For this review, use the dimensioned drawing (mm, ordinates from the lowest corner) and the shaded views. A direction names the side the tool comes from. Round coordinates to 2 decimals unless told otherwise and drop trailing zeros. Loops run counter-clockwise (first coordinate to the right, second up) from the corner with the lowest first, then second, coordinate; pieces in that order, holes last. Notation, with made-up numbers: (-11, 9.5) -> (21, 9.5) arc R23 cw to (21, 32.5) -> close; hole circle Ø3 at (49.5, 30.5). An arc over 180 degrees is marked (long way). Write each question's results on one line, items separated by ' | '.
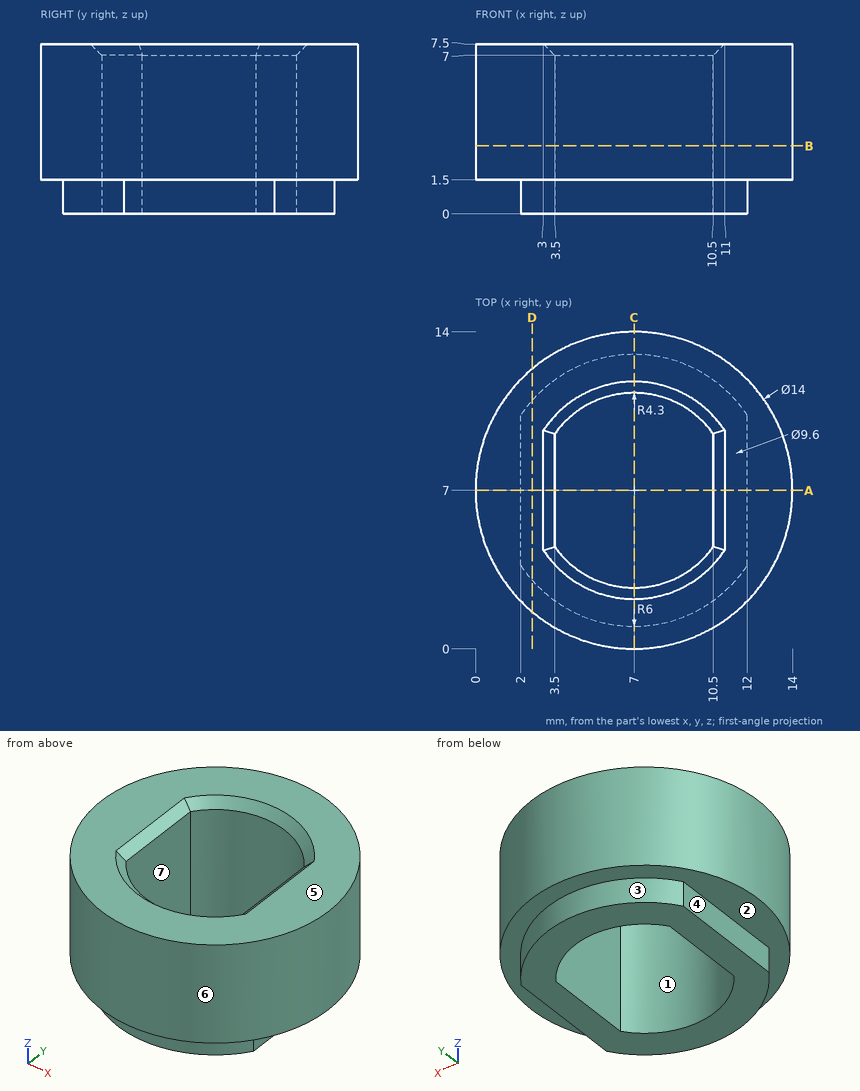
1. Consider section A-A (y = 7). State the section outline as (x, z) points.
Values found:
outline: (0, 1.5) -> (2, 1.5) -> (2, 0) -> (3.5, 0) -> (3.5, 7) -> (3, 7.5) -> (0, 7.5) -> close; (10.5, 0) -> (12, 0) -> (12, 1.5) -> (14, 1.5) -> (14, 7.5) -> (11, 7.5) -> (10.5, 7) -> close
2. For pin 1 (1.5 mm diameter, centred on y = 8, z = 3, fed in from +X); pin 2 (1.6 mm diameter, centred on y = 6.5, z = 0.5, fed in from -X); pin 3 (4 mm diameter, centred on x = 9.5, z = 6, fed in from +Y), all flat-tipped, find the tip position at first contact; note any pin that passes through.
Values found:
pin 1: stops at x = 14 | pin 2: stops at x = 2 | pin 3: stops at y = 13.98
3. Draft analysis for pull direction X (two halves, no side actions). For the marked faces 4, 5, 6 and 7, state which applies: released by +X, released by -X, zero draft, split by the parting line, or undercut.
Values found:
face 4: released by -X | face 5: zero draft | face 6: split by the parting line | face 7: undercut
4. To check wall thickness, follow probe 1 along X at (y, z) = (5.75, 1.25); probe 2 along Z at (x, y) = (1, 3.5); probe 3 along X at (y, z) = (12, 1.25). State the ranges of each line that lie inside material, in increasing order.
Values found:
probe 1: x = 2 to 3.5, 10.5 to 12 | probe 2: z = 1.5 to 7.5 | probe 3: x = 3.68 to 10.32
5. Tool access review of the marked faces 1, 2 and 3: name each direction out of +Z, -Z, +X, -X, +Y, -Y from which nothing blocks a thin tool from reaching the whole face with its end or side.
Values found:
face 1: +Z, -Z | face 2: -Z | face 3: -Z, +Y
6. Consider section B-B (z = 3). State the section outline as (x, y) points.
Values found:
outline: circle Ø14 at (7, 7); hole (3.5, 4.5) arc R4.3 ccw to (10.5, 4.5) -> (10.5, 9.5) arc R4.3 ccw to (3.5, 9.5) -> close
7. Consider section C-C (x = 7). State the section outline as (y, z) points, plus the area to 4 significant figures.
Values found:
outline: (0, 1.5) -> (1, 1.5) -> (1, 0) -> (2.7, 0) -> (2.7, 7) -> (2.2, 7.5) -> (0, 7.5) -> close; (11.3, 0) -> (13, 0) -> (13, 1.5) -> (14, 1.5) -> (14, 7.5) -> (11.8, 7.5) -> (11.3, 7) -> close | area: 37.25 mm2
8. Consider section D-D (x = 2.5). State the section outline as (y, z) points.
Values found:
outline: (1.64, 1.5) -> (3.03, 1.5) -> (3.03, 0) -> (10.97, 0) -> (10.97, 1.5) -> (12.36, 1.5) -> (12.36, 7.5) -> (1.64, 7.5) -> close
